Read the model definition and answer for the solid it produces. Units are mm, in the model's axes. A direction names the side the tool comes from. Give positions to 0.01 mm unless a question says otherwise; leave off trailing zeros. Order: outer loops, then holes, each group sorted by start corner. A loop starts at its lowest first (then second) coordinate and runs counter-clockwise, first axis right, second up.
```python
from build123d import *

# Parameters (mm, degrees)
F2_DEPTH  = 18.5
F3_R      = 1.55
F4_DEPTH  = 3.075
F5_W      = 6
F5_H      = 0.5
F6_DEPTH  = 0.1
F5_W_2    = 4
F5_H_2    = 2.25
F7_DEPTH  = 0.6
F8_W      = 4
F8_H      = 0.5
F9_DEPTH  = 0.9
F8_H_2    = 0.47
F10_DEPTH = 0.1
F11_W     = 4
F11_H     = 0.5
F12_DEPTH = 0.9
F11_H_2   = 0.47
F13_DEPTH = 0.1
F14_W     = 4
F14_H     = 0.5
F15_DEPTH = 0.7
F16_W     = 8
F16_H     = 7
F17_DEPTH = 1
F17_TAPER = 45
F18_W     = 8
F18_H     = 7
F19_DEPTH = 1
F19_TAPER = 45
F22_DEPTH = 0.2
F23_ANGLE = 90


with BuildPart() as f2:
    # F1 (on Front) → F2 (new body)
    with BuildSketch(Plane.XZ):
        with BuildLine():
            Line((-33.5725, -6), (33.5725, -6))
            ThreePointArc((33.5725, -6), (34.6331601718, -5.5606601718), (35.0725, -4.5))
            Line((35.0725, -4.5), (35.0725, 4.5))
            ThreePointArc((35.0725, 4.5), (34.6331601718, 5.5606601718), (33.5725, 6))
            Line((33.5725, 6), (-33.5725, 6))
            ThreePointArc((-33.5725, 6), (-34.6331601718, 5.5606601718), (-35.0725, 4.5))
            Line((-35.0725, 4.5), (-35.0725, -4.5))
            ThreePointArc((-35.0725, -4.5), (-34.6331601718, -5.5606601718), (-33.5725, -6))
        make_face()
        with BuildLine():
            ThreePointArc((-14.9225, -0.925), (-15.5082864376, -2.3392135624), (-16.9225, -2.925))
            Line((-16.9225, -2.925), (-30.0725, -2.925))
            ThreePointArc((-30.0725, -2.925), (-31.4867135624, -2.3392135624), (-32.0725, -0.925))
            Line((-32.0725, -0.925), (-32.0725, 0.925))
            ThreePointArc((-32.0725, 0.925), (-31.4867135624, 2.3392135624), (-30.0725, 2.925))
            Line((-30.0725, 2.925), (-16.9225, 2.925))
            ThreePointArc((-16.9225, 2.925), (-15.5082864376, 2.3392135624), (-14.9225, 0.925))
            Line((-14.9225, 0.925), (-14.9225, -0.925))
        make_face(mode=Mode.SUBTRACT)
        with BuildLine():
            Line((-9.6675, 4.65), (-1.0875, 4.65))
            ThreePointArc((-1.0875, 4.65), (-0.0268398282, 4.2106601718), (0.4125, 3.15))
            Line((0.4125, 3.15), (0.4125, -3.15))
            ThreePointArc((0.4125, -3.15), (-0.0268398282, -4.2106601718), (-1.0875, -4.65))
            Line((-1.0875, -4.65), (-9.6675, -4.65))
            ThreePointArc((-9.6675, -4.65), (-10.7281601718, -4.2106601718), (-11.1675, -3.15))
            Line((-11.1675, -3.15), (-11.1675, 3.15))
            ThreePointArc((-11.1675, 3.15), (-10.7281601718, 4.2106601718), (-9.6675, 4.65))
        make_face(mode=Mode.SUBTRACT)
        with BuildLine():
            Line((4.3325, 4.215), (12.9125, 4.215))
            ThreePointArc((12.9125, 4.215), (13.9731601718, 3.7756601718), (14.4125, 2.715))
            Line((14.4125, 2.715), (14.4125, -2.715))
            ThreePointArc((14.4125, -2.715), (13.9731601718, -3.7756601718), (12.9125, -4.215))
            Line((12.9125, -4.215), (4.3325, -4.215))
            ThreePointArc((4.3325, -4.215), (3.2718398282, -3.7756601718), (2.8325, -2.715))
            Line((2.8325, -2.715), (2.8325, 2.715))
            ThreePointArc((2.8325, 2.715), (3.2718398282, 3.7756601718), (4.3325, 4.215))
        make_face(mode=Mode.SUBTRACT)
        with BuildLine():
            ThreePointArc((32.0725, -3.8), (32.0139213562, -3.9414213562), (31.8725, -4))
            Line((31.8725, -4), (17.0725, -4))
            ThreePointArc((17.0725, -4), (16.9310786438, -3.9414213562), (16.8725, -3.8))
            Line((16.8725, -3.8), (16.8725, 3.8))
            ThreePointArc((16.8725, 3.8), (16.9310786438, 3.9414213562), (17.0725, 4))
            Line((17.0725, 4), (31.8725, 4))
            ThreePointArc((31.8725, 4), (32.0139213562, 3.9414213562), (32.0725, 3.8))
            Line((32.0725, 3.8), (32.0725, -3.8))
        make_face(mode=Mode.SUBTRACT)
    extrude(amount=-F2_DEPTH)

    # F3 (on face) → F4 (cut, through all)
    with BuildSketch(Plane.XY.offset(6)):
        with Locations((-23.4975, 13.2)):
            Circle(F3_R)
    extrude(amount=-F4_DEPTH, mode=Mode.SUBTRACT)

    # F5 (on face) → F6 (join)
    with BuildSketch(Plane.XY.offset(-2.925)):
        with Locations((-23.4975, 18.25)):
            Rectangle(F5_W, F5_H)
    extrude(amount=F6_DEPTH)

    # F5 (on face) → F7 (join)
    with BuildSketch(Plane.XY.offset(-2.925)):
        with Locations((-23.4975, 6.575)):
            Rectangle(F5_W_2, F5_H_2)
    extrude(amount=F7_DEPTH)

    # F8 (on face) → F9 (join)
    with BuildSketch(Plane.XY.offset(-4.65)):
        with Locations((-5.3775, 18.25)):
            Rectangle(F8_W, F8_H)
    extrude(amount=F9_DEPTH)

    # F8 (on face) → F10 (join)
    with BuildSketch(Plane.XY.offset(-4.65)):
        with Locations((-5.3775, 0.235)):
            Rectangle(F8_W, F8_H_2)
    extrude(amount=F10_DEPTH)

    # F11 (on face) → F12 (join)
    with BuildSketch(Plane.XY.offset(-4.215)):
        with Locations((8.6225, 18.25)):
            Rectangle(F11_W, F11_H)
    extrude(amount=F12_DEPTH)

    # F11 (on face) → F13 (join)
    with BuildSketch(Plane.XY.offset(-4.215)):
        with Locations((8.6225, 0.235)):
            Rectangle(F11_W, F11_H_2)
    extrude(amount=F13_DEPTH)

    # F14 (on face) → F15 (join)
    with BuildSketch(Plane.XY.offset(-4)):
        with Locations((24.4725, 18.25)):
            Rectangle(F14_W, F14_H)
    extrude(amount=F15_DEPTH)

    # F16 (on face) → F17 (cut)
    with BuildSketch(Plane.YZ.offset(35.0725)):
        with Locations((9.25, 0)):
            Rectangle(F16_W, F16_H)
    extrude(amount=-F17_DEPTH, taper=F17_TAPER, mode=Mode.SUBTRACT)

    # F18 (on face) → F19 (cut)
    with BuildSketch(Plane(origin=(-35.0725, 0, 0), x_dir=(0, -1, 0), z_dir=(-1, 0, 0))):
        with Locations((-9.25, 0)):
            Rectangle(F18_W, F18_H)
    extrude(amount=-F19_DEPTH, taper=F19_TAPER, mode=Mode.SUBTRACT)

    # F21 (on face) → F22 (join)
    with BuildSketch(Plane(origin=(0, 18.5, 0), x_dir=(-1, 0, 0), z_dir=(0, 1, 0))):
        with BuildLine():
            Line((-33.5725, 6), (-31.6655044446, 6))
            ThreePointArc((-31.6655044446, 6), (-36.7544805153, 7.6819805153), (-35.0725, 2.5930044446))
            Line((-35.0725, 2.5930044446), (-35.0725, 4.5))
            ThreePointArc((-35.0725, 4.5), (-34.6331601718, 5.5606601718), (-33.5725, 6))
        make_face()
        with BuildLine():
            Line((-35.0725, -4.5), (-35.0725, -2.5930044446))
            ThreePointArc((-35.0725, -2.5930044446), (-36.7544805153, -7.6819805153), (-31.6655044446, -6))
            Line((-31.6655044446, -6), (-33.5725, -6))
            ThreePointArc((-33.5725, -6), (-34.6331601718, -5.5606601718), (-35.0725, -4.5))
        make_face()
        with BuildLine():
            ThreePointArc((37.6331601718, 5.5606601718), (34.8534245792, 8.5525631767), (31.6655044446, 6))
            Line((31.6655044446, 6), (33.5725, 6))
            ThreePointArc((33.5725, 6), (34.6331601718, 5.5606601718), (35.0725, 4.5))
            Line((35.0725, 4.5), (35.0725, 2.5930044446))
            ThreePointArc((35.0725, 2.5930044446), (36.9045055313, 3.6008157245), (37.6331601718, 5.5606601718))
        make_face()
        with BuildLine():
            ThreePointArc((37.6331601718, -5.5606601718), (36.9045055313, -3.6008157245), (35.0725, -2.5930044446))
            Line((35.0725, -2.5930044446), (35.0725, -4.5))
            ThreePointArc((35.0725, -4.5), (34.6331601718, -5.5606601718), (33.5725, -6))
            Line((33.5725, -6), (31.6655044446, -6))
            ThreePointArc((31.6655044446, -6), (34.8534245792, -8.5525631767), (37.6331601718, -5.5606601718))
        make_face()
    extrude(amount=-F22_DEPTH)


with BuildPart() as f2_1:
    # F23: moved
    add(f2.part.rotate(Axis((0, 18.5, 6), (-1, 0, 0)), F23_ANGLE))


solid = f2_1.part
```
1) The part is cut by section B-B on z = 16. Count the separate pieces of the cut face and the enclosed holes in it, and give its area (3 significant figures).
Final values:
separate pieces: 1
enclosed holes: 4
area: 408 mm2
2) The part is cut by section A-A on x = 12. Determine the outline of the cut face in (y, z) (3 decimals).
Final values:
outline: (6.5, 6) - (8.285, 6) - (8.285, 24.5) - (6.5, 24.5) - close; (16.715, 6) - (18.5, 6) - (18.5, 24.5) - (16.715, 24.5) - close
3) Consider L1, parallel to Y at x = 29, z = 7; L2, parallel to Y at x = -26, z = 17.25 (3 decimals); L3, parallel to X at y = 13, z = 14.5. Determine where each line is inside the solid, lowest interval first.
Final values:
L1: y = 6.5 to 8.5, 16.5 to 18.5
L2: y = 6.5 to 9.575, 15.425 to 18.5
L3: x = -34.07 to -32.07, -14.92 to -11.17, 0.41 to 2.83, 14.41 to 16.87, 32.07 to 34.07
4) For a pull along X with two mould halves and no side action, classify faces 5 (the face through (-15.52, 14.85, 15.38)), 6 (the face through (35, 19, 6.2)), 7 (the face through (-34.621, 18.072, 15.478)) as released by +X, released by -X, zero draft, split by the parting line, or undercut.
Final values:
face 5: undercut
face 6: zero draft
face 7: released by -X
5) A tool of negligible diameter and unlimited length cuts with its end or side. For faces 1 (the face through (-11.168, 12, 15)), 2 (the face through (9, 8.285, 15)), 3 (the face through (-35, 19, 6.2)), 4 (the face through (25, 8.5, 15)), from which of +Z, -Z, +X, -X, +Y, -Y can it reach the whole face along a straight path? Write none if from no direction.
Final values:
face 1: +Z, -Z
face 2: none
face 3: +Z, -X, +Y
face 4: +Z
6) Given pin 1 (8 mm diameter, centred on y = 15.5, z = 16, fed in from +X); pin 2 (1.5 mm diameter, centred on x = 3.5, z = 15.5, fed in from +Y); pin 3 (1.6 mm diameter, centred on y = 11, z = 18, fed in from -X); pin 4 (6.5 mm diameter, centred on x = -34, y = 5.5, fed in from +Z), each flat-ended and moving along its own axis, determine where each tip first touches the part or whether it passes through.
Final values:
pin 1: stops at x = 35.07
pin 2: stops at y = 18.5
pin 3: stops at x = -34.62
pin 4: stops at z = 24.5
